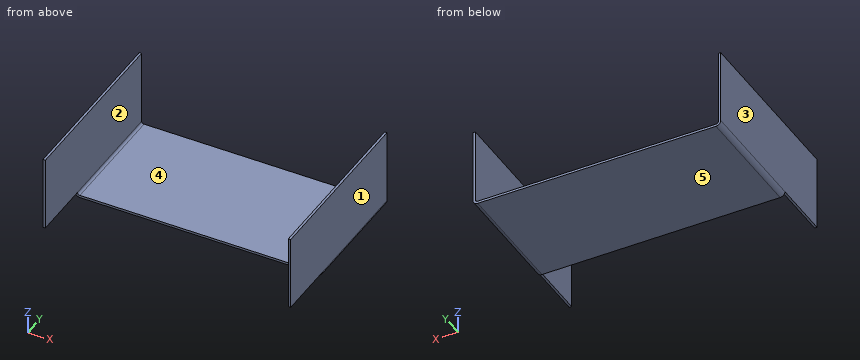
Autodesk Inventor part; units mm, degrees
ref_plane "YZ Plane" through (0, 0, 0) normal (1, 0, 0) x (0, 1, 0)
ref_plane "XZ Plane" through (0, 0, 0) normal (0, 1, 0) x (-1, 0, 0)
ref_plane "XY Plane" through (0, 0, 0) normal (0, 0, 1) x (1, 0, 0)
sketch "Sketch1" plane through (0, 0, 0) normal (0, 0, 1) x (1, 0, 0)
  line L0 (0, 0) -> (317.5, 0)
  line L1 (317.5, 0) -> (317.5, 152.4)
  line L2 (317.5, 152.4) -> (0, 152.4)
  line L3 (0, 152.4) -> (0, 0)
  dimension "d0" = 317.5
  dimension "d1" = 152.4
extrude "Plate1" add sketch "Sketch1" along normal blind 3.048
sketch "Sketch2" plane through (3.048, 0, 0) normal (-1, 0, 0) x (0, -1, 0)
  line L0 (-152.4, 0) -> (0, 0)
  line L1 (0, 0) -> (0, 101.6)
  line L2 (0, 101.6) -> (-152.4, 101.6)
  line L3 (-152.4, 101.6) -> (-152.4, 0)
edge flange "Flange1" height 101.6 angle 90 thickness 3.048 bend radius 3.048 thickness toward (-1, 0, 0) relief tear relief width 3.048 relief depth 1.524 corner gap 3.048 corner form 0 edges at (0, 76.2, 3.048) (317.5, 76.2, 3.048) wall of the first edge with corners at (3.048, 152.4, 0) (3.048, 0, 0) (3.048, 0, 101.6) (3.048, 152.4, 101.6)
bend "Bend1"
corner "Corner1"
sketch "Sketch3" plane through (0, 0, 101.6) normal (0, -1, 0) x (1, 0, 0)
  line L0 (0, -95.504) -> (3.048, -95.504)
  line L1 (3.048, 0) -> (3.048, -95.504)
  line L2 (3.048, 0) -> (0, 0)
  line L3 (0, 0) -> (0, -95.504)
  line L4 (314.452, -95.504) -> (317.5, -95.504)
  line L5 (317.5, -95.504) -> (317.5, 0)
  line L6 (314.452, 0) -> (317.5, 0)
  line L7 (314.452, 0) -> (314.452, -95.504)
  point P0 (0, -101.6)
extrude "Extrusion1" add sketch "Sketch3" along normal blind 76.2
equation "\"d3\" = BendReliefWidth"
equation "\"d4\" = BendReliefDepth"
equation "\"d5\" = MinimumRemnant"
equation "\"d6\" = BendRadius"
equation "\"d9\" = BendRadius"
equation "\"d10\" = CornerReliefSize"
equation "\"d11\" = GapSize"
equation "\"d12\" = JacobiRadiusSize"
equation "\"BendRadius\" = Thickness"
equation "\"BendReliefWidth\" = Thickness"
equation "\"BendReliefDepth\" = 0.5 * Thickness"
equation "\"CornerReliefSize\" = 4 * Thickness"
equation "\"MinimumRemnant\" = 2 * Thickness"
equation "\"TransitionRadius\" = BendRadius"
equation "\"JacobiRadiusSize\" = BendRadius"
equation "\"GapSize\" = Thickness"
equation "\"d2\" = BendRadius"
properties part number "Chute(2)"
Could you check a few things on this model? Use its own coordinates, in mm. Face numbers are marked on the shaded views. A direction names the side the tool comes from. Coordinates: 2 decimals unless noted, no trailing zeros. Order: outer loops, then holes, each group sorted by start corner. A loop starts at its lowest first (then second) coordinate and runs counter-clockwise, first axis right, second up. Notation, with made-up numbers: M -27,-24.5 L -8,-24.5 A25 cw -8,11.5 Z; hole C 13,11 d3. An arc over 180 degrees is marked long. Use one line per item in the form item = value. Start each with the question number.
1. Please list where these lines run through material, in increasing order: line 1 (X direction, y = 116, z = 89); line 2 (Z direction, x = 227, y = 143.5).
2. Suppose I cut it at C-C on y = 64.5. Write out the boundary of the cut face in (x, z).
3. On a 3-axis mill with a long thin cutter (end or side, diameter ignored), from which of +Z, -Z, +X, -X, +Y, -Y can I reach the whole of each face in a straight line? I mean the marked faces 4 and 5. Say none if no direction works.
4. We'd pull the mould along X, two halves only. Please class the marked faces 1, 2 and 3: +X half, -X half, draft (parallel to the pull), parting line (faces both ways), or undercut.
5. Suppose I cut it at B-B on y = -22.5. Write out the boundary of the cut face in (x, z).
6. For pin 1 (3 mm diameter, centred on y = 57.5, z = 12.5, fed in from -X); pin 2 (3.5 mm diameter, centred on x = 1, y = -33.5, fed in from -Z); pin 3 (3 mm diameter, centred on x = 236, z = 2.5, fed in from -Y), each with a flat end and sliding along its axis, tell me the tip position at first contact or that it passes through.
7. Suppose I cut it at A-A on z = 81.5. Write out the boundary of the cut face in (x, y), then the cut area to 3 significant figures.
8. Suppose I cut it at D-D on x = 89. Write out the boundary of the cut face in (y, z).
Geometry says:
q1.line_1 = 0 to 3.05, 314.45 to 317.5
q1.line_2 = 0 to 3.05
q2.outline = M 0,6.1 A6.1 ccw 6.1,0 L 311.4,0 A6.1 ccw 317.5,6.1 L 317.5,101.6 L 314.45,101.6 L 314.45,6.1 A3.05 cw 311.4,3.05 L 6.1,3.05 A3.05 cw 3.05,6.1 L 3.05,101.6 L 0,101.6 Z
q3.face_4 = +Z, +Y, -Y
q3.face_5 = -Z, +X, -X, +Y, -Y
q4.face_1 = +X half
q4.face_2 = undercut
q4.face_3 = -X half
q5.outline = M 0,6.1 L 3.05,6.1 L 3.05,101.6 L 0,101.6 Z; M 314.45,6.1 L 317.5,6.1 L 317.5,101.6 L 314.45,101.6 Z
q6.pin_1 = 0
q6.pin_2 = 6.1
q6.pin_3 = 0
q7.outline = M 0,-76.2 L 3.05,-76.2 L 3.05,152.4 L 0,152.4 Z; M 314.45,-76.2 L 317.5,-76.2 L 317.5,152.4 L 314.45,152.4 Z
q7.area = 1,390 mm^2
q8.outline = M 0,0 L 152.4,0 L 152.4,3.05 L 0,3.05 Z
